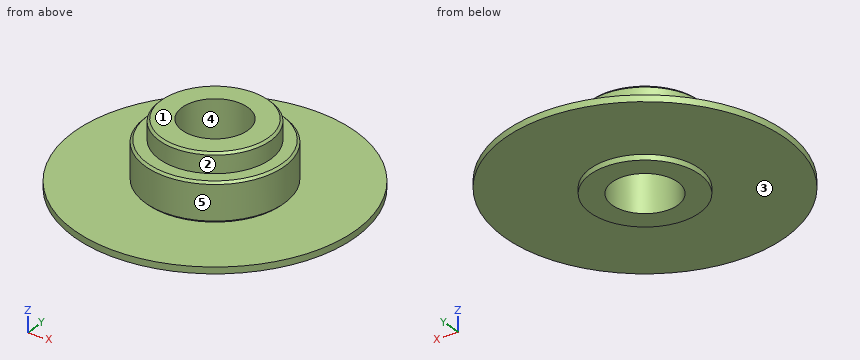
from build123d import *

# Parameters (mm, degrees)
SKETCH1_R           = 5.08
BOSS_EXTRUDE1_DEPTH = 1.8
SKETCH2_R           = 6.35
BOSS_EXTRUDE2_DEPTH = 3.56
CHAMFER1_SIZE       = 0.2
SKETCH3_R           = 12.85
BOSS_EXTRUDE3_DEPTH = 0.59
SKETCH4_R           = 5
BOSS_EXTRUDE4_DEPTH = 0.5
SKETCH5_R           = 3
CUT_EXTRUDE1_DEPTH  = 7.45


with BuildPart() as part:
    # Sketch1 → Boss-Extrude1 (new body)
    with BuildSketch(Plane.XY):
        Circle(SKETCH1_R)
    extrude(amount=-BOSS_EXTRUDE1_DEPTH)

    # Sketch2 → Boss-Extrude2 (add)
    with BuildSketch(Plane(origin=(0, 0, -1.8), x_dir=(-1, 0, 0), z_dir=(0, 0, -1))):
        Circle(SKETCH2_R)
    extrude(amount=BOSS_EXTRUDE2_DEPTH)

    # Chamfer1
    chamfer1_edges = [part.edges().sort_by_distance(p)[0] for p in [
        (-5.08, 0, 0),
        (6.35, 0, -1.8),
        (6.35, 0, -5.36),
    ]]
    chamfer(chamfer1_edges, length=CHAMFER1_SIZE)

    # Sketch3 → Boss-Extrude3 (add)
    with BuildSketch(Plane(origin=(0, 0, -5.36), x_dir=(-1, 0, 0), z_dir=(0, 0, -1))):
        Circle(SKETCH3_R)
    extrude(amount=BOSS_EXTRUDE3_DEPTH)

    # Sketch4 → Boss-Extrude4 (add)
    with BuildSketch(Plane(origin=(0, 0, -5.95), x_dir=(-1, 0, 0), z_dir=(0, 0, -1))):
        Circle(SKETCH4_R)
    extrude(amount=BOSS_EXTRUDE4_DEPTH)

    # Sketch5 → Cut-Extrude1 (cut, through all)
    with BuildSketch(Plane.XY):
        Circle(SKETCH5_R)
    extrude(amount=-CUT_EXTRUDE1_DEPTH, mode=Mode.SUBTRACT)


solid = part.part
Verification items for the finished model (mm, model axes). Face numbers are marked on the shaded views. A direction names the side the tool comes from. Round coordinates to 2 decimals unless told otherwise and drop trailing zeros. Order: outer loops, then holes, each group sorted by start corner. A loop starts at its lowest first (then second) coordinate and runs counter-clockwise, first axis right, second up. Notation, with made-up numbers: (72, 75) -> (81, 75) arc R19 cw to (81, 94) -> close; hole circle Ø6 at (62, 50.5). An arc over 180 degrees is marked (long way). Put each result on its own line as item: value.
1) Section check C-C (z = -3.5). Record the cut outline in (x, y), then the cut area to 3 significant figures.
Final values:
outline: circle Ø12.7 at (0, 0); hole circle Ø6 at (0, 0)
area: 98.4 mm^2
2) Set-up check for the marked faces 1 and 2: record each of +Z, -Z, +X, -X, +Y, -Y from which the full face is reachable in a straight line by a thin tool's end or side.
Final values:
face 1: +Z, +X, -X, +Y, -Y
face 2: +Z
3) Section check A-A (x = 0). Record the cut outline in (y, z), then the cut area to 3 significant figures.
Final values:
outline: (-12.85, -5.95) -> (-5, -5.95) -> (-5, -6.45) -> (-3, -6.45) -> (-3, 0) -> (-4.88, 0) -> (-5.08, -0.2) -> (-5.08, -1.8) -> (-6.15, -1.8) -> (-6.35, -2) -> (-6.35, -5.16) -> (-6.15, -5.36) -> (-12.85, -5.36) -> close; (3, -6.45) -> (5, -6.45) -> (5, -5.95) -> (12.85, -5.95) -> (12.85, -5.36) -> (6.15, -5.36) -> (6.35, -5.16) -> (6.35, -2) -> (6.15, -1.8) -> (5.08, -1.8) -> (5.08, -0.2) -> (4.88, 0) -> (3, 0) -> close
area: 44.8 mm^2
4) Depth check by flat-ended pin: pin 1 (10 mm diameter, centred on x = -3, y = -0.5, fed in from +Z); pin 2 (1.5 mm diameter, centred on x = 8.5, y = 4.5, fed in from -Z); pin 3 (5 mm diameter, centred on x = 1, y = -8, fed in from +Z); pin 4 (1.5 mm diameter, centred on y = 3.5, z = -1, fed in from +X). Enter the tip coordinate at first touch or a pass-through.
Final values:
pin 1: stops at z = 0
pin 2: stops at z = -5.95
pin 3: stops at z = -1.8
pin 4: stops at x = 4.27
5) Mould release check, pull along Y, two halves, no side actions. Record for the marked faces 3, 4 and 5: +Y half, -Y half, draft (parallel to the pull), parting line (faces both ways), or undercut.
Final values:
face 3: draft
face 4: undercut
face 5: parting line
6) Material ranges on line 1 (Y direction, x = 0, z = -4.25); line 2 (Z direction, x = 7, y = 6.5); line 3 (X direction, y = -2.5, z = -5), recorded low to high.
Final values:
line 1: y = -6.35 to -3, 3 to 6.35
line 2: z = -5.95 to -5.36
line 3: x = -5.84 to -1.66, 1.66 to 5.84
7) Section check D-D (y = -7.5). Record the cut outline in (x, z).
Final values:
outline: (-10.43, -5.95) -> (10.43, -5.95) -> (10.43, -5.36) -> (-10.43, -5.36) -> close
